Input: part model. Units: mm. Frame: model coordinates. Give positions to 0.01 mm unless a question says otherwise; leave off trailing zeros. Loops run counter-clockwise (first coordinate to the right, second up) from the corner with the lowest first, then second, coordinate; pieces in that order, holes last.
from build123d import *

# Parameters (mm, degrees)
CYLINDER013_R          = 0.565
CYLINDER013_DEPTH      = 5
CYLINDER012_R          = 0.565
CYLINDER012_DEPTH      = 5
CYLINDER008_R          = 0.565
CYLINDER008_DEPTH      = 5
CYLINDER003_R          = 0.565
CYLINDER003_DEPTH      = 5
BOX018_W               = 0.4
BOX018_H               = 1
BOX018_DEPTH           = 1
BOX018_PLACEMENT_ANGLE = 90
BOX001_W               = 0.4
BOX001_H               = 1
BOX001_DEPTH           = 1
BOX001_PLACEMENT_ANGLE = 90
BOX014_W               = 0.4
BOX014_H               = 1
BOX014_DEPTH           = 1
BOX014_PLACEMENT_ANGLE = 90
BOX015_W               = 0.4
BOX015_H               = 1
BOX015_DEPTH           = 1
BOX015_PLACEMENT_ANGLE = 90
BOX017_W               = 0.4
BOX017_H               = 1
BOX017_DEPTH           = 1
BOX016_W               = 0.4
BOX016_H               = 1
BOX016_DEPTH           = 1
BOX013_W               = 0.4
BOX013_H               = 1
BOX013_DEPTH           = 1
BOX_W                  = 0.4
BOX_H                  = 1
BOX_DEPTH              = 1
BOX012_W               = 11
BOX012_H               = 11
BOX012_DEPTH           = 0.3
CHAMFER002_SIZE        = 0.5
CUT010_PLACEMENT_ANGLE = 90


with BuildPart() as cilindro009:
    # Cylinder013 → Cylinder013 (new body)
    with BuildSketch(Plane(origin=(4.2, -4.2, 0), x_dir=(1, 0, 0), z_dir=(0, 0, 1))):
        Circle(CYLINDER013_R)
    extrude(amount=CYLINDER013_DEPTH)


with BuildPart() as cilindro008:
    # Cylinder012 → Cylinder012 (new body)
    with BuildSketch(Plane(origin=(-4.2, -4.2, 0), x_dir=(1, 0, 0), z_dir=(0, 0, 1))):
        Circle(CYLINDER012_R)
    extrude(amount=CYLINDER012_DEPTH)


with BuildPart() as cilindro006:
    # Cylinder008 → Cylinder008 (new body)
    with BuildSketch(Plane(origin=(4.2, 4.2, 0), x_dir=(1, 0, 0), z_dir=(0, 0, 1))):
        Circle(CYLINDER008_R)
    extrude(amount=CYLINDER008_DEPTH)


with BuildPart() as cilindro007:
    # Cylinder003 → Cylinder003 (new body)
    with BuildSketch(Plane(origin=(-4.2, 4.2, 0), x_dir=(1, 0, 0), z_dir=(0, 0, 1))):
        Circle(CYLINDER003_R)
    extrude(amount=CYLINDER003_DEPTH)


with BuildPart() as obj1:
    # Box018 → Box018 (new body)
    with BuildSketch(Plane.XY):
        with Locations((0.2, 0.5)):
            Rectangle(BOX018_W, BOX018_H)
    extrude(amount=BOX018_DEPTH)


with BuildPart() as obj1_1:
    # Box018 placement: moved
    add(obj1.part.moved(Location((6.3, -3, 3))).rotate(Axis((6.3, -3, 3), (0, 0, 1)), BOX018_PLACEMENT_ANGLE))


with BuildPart() as obj2:
    # Box001 → Box001 (new body)
    with BuildSketch(Plane.XY):
        with Locations((0.2, 0.5)):
            Rectangle(BOX001_W, BOX001_H)
    extrude(amount=BOX001_DEPTH)


with BuildPart() as obj2_1:
    # Box001 placement: moved
    add(obj2.part.moved(Location((6.3, 2.5, 3))).rotate(Axis((6.3, 2.5, 3), (0, 0, 1)), BOX001_PLACEMENT_ANGLE))


with BuildPart() as obj3:
    # Box014 → Box014 (new body)
    with BuildSketch(Plane.XY):
        with Locations((0.2, 0.5)):
            Rectangle(BOX014_W, BOX014_H)
    extrude(amount=BOX014_DEPTH)


with BuildPart() as obj3_1:
    # Box014 placement: moved
    add(obj3.part.moved(Location((-5.3, -3, 3))).rotate(Axis((-5.3, -3, 3), (0, 0, 1)), BOX014_PLACEMENT_ANGLE))


with BuildPart() as obj4:
    # Box015 → Box015 (new body)
    with BuildSketch(Plane.XY):
        with Locations((0.2, 0.5)):
            Rectangle(BOX015_W, BOX015_H)
    extrude(amount=BOX015_DEPTH)


with BuildPart() as obj4_1:
    # Box015 placement: moved
    add(obj4.part.moved(Location((-5.3, 2.5, 3))).rotate(Axis((-5.3, 2.5, 3), (0, 0, 1)), BOX015_PLACEMENT_ANGLE))


with BuildPart() as obj5:
    # Box017 → Box017 (new body)
    with BuildSketch(Plane(origin=(3, -6.2, 3), x_dir=(1, 0, 0), z_dir=(0, 0, 1))):
        with Locations((0.2, 0.5)):
            Rectangle(BOX017_W, BOX017_H)
    extrude(amount=BOX017_DEPTH)


with BuildPart() as obj6:
    # Box016 → Box016 (new body)
    with BuildSketch(Plane(origin=(-3, -6.2, 3), x_dir=(1, 0, 0), z_dir=(0, 0, 1))):
        with Locations((0.2, 0.5)):
            Rectangle(BOX016_W, BOX016_H)
    extrude(amount=BOX016_DEPTH)


with BuildPart() as obj7:
    # Box013 → Box013 (new body)
    with BuildSketch(Plane(origin=(3, 5.2, 3), x_dir=(1, 0, 0), z_dir=(0, 0, 1))):
        with Locations((0.2, 0.5)):
            Rectangle(BOX013_W, BOX013_H)
    extrude(amount=BOX013_DEPTH)


with BuildPart() as obj8:
    # Box → Box (new body)
    with BuildSketch(Plane(origin=(-3, 5.2, 3), x_dir=(1, 0, 0), z_dir=(0, 0, 1))):
        with Locations((0.2, 0.5)):
            Rectangle(BOX_W, BOX_H)
    extrude(amount=BOX_DEPTH)


with BuildPart() as obj9:
    # Box012 → Box012 (new body)
    with BuildSketch(Plane(origin=(-5.5, -5.5, 3.6), x_dir=(1, 0, 0), z_dir=(0, 0, 1))):
        with Locations((5.5, 5.5)):
            Rectangle(BOX012_W, BOX012_H)
    extrude(amount=BOX012_DEPTH)

    # Chamfer002
    chamfer002_edges = [obj9.edges().sort_by_distance(p)[0] for p in [
        (-5.5, -5.5, 3.75),
        (-5.5, 5.5, 3.75),
        (5.5, -5.5, 3.75),
        (5.5, 5.5, 3.75),
    ]]
    chamfer(chamfer002_edges, length=CHAMFER002_SIZE)


with BuildPart() as obj9_1:
    # Chamfer002 placement: moved
    add(obj9.part.moved(Location((0, 0, -0.4))))

    # Cut021: cut obj8
    add(obj8.part, mode=Mode.SUBTRACT)

    # Cut022: cut obj7
    add(obj7.part, mode=Mode.SUBTRACT)

    # Cut029: cut obj6
    add(obj6.part, mode=Mode.SUBTRACT)

    # Cut006: cut obj5
    add(obj5.part, mode=Mode.SUBTRACT)

    # Cut005: cut obj4
    add(obj4_1.part, mode=Mode.SUBTRACT)

    # Cut023: cut obj3
    add(obj3_1.part, mode=Mode.SUBTRACT)

    # Cut009: cut obj2
    add(obj2_1.part, mode=Mode.SUBTRACT)

    # Cut003: cut obj1
    add(obj1_1.part, mode=Mode.SUBTRACT)

    # Cut028: cut Cilindro007
    add(cilindro007.part, mode=Mode.SUBTRACT)

    # Cut027: cut Cilindro006
    add(cilindro006.part, mode=Mode.SUBTRACT)

    # Cut004: cut Cilindro008
    add(cilindro008.part, mode=Mode.SUBTRACT)

    # Cut010: cut Cilindro009
    add(cilindro009.part, mode=Mode.SUBTRACT)


with BuildPart() as obj9_2:
    # Cut010 placement: moved
    add(obj9_1.part.moved(Location((0, 1.7, 1.6))).rotate(Axis((0, 1.7, 1.6), (0, 0, 1)), CUT010_PLACEMENT_ANGLE))


solid = obj9_2.part
(1) Pin query (flat end, axial travel): pin 1 Ø1.5 at (x, y) = (-4.2, -2.5) entering from -Z. Return the tip coordinate at first contact, or that it passes through.
Values follow:
pin 1: stops at z = 4.8
(2) Ray query, probe 1 along X at (y, z) = (-2.5, 5) (3 decimals); probe 2 along Y at (x, z) = (4.25, 4.9); probe 3 along Y at (x, z) = (5.25, 4.85). Return the intervals inside material, ascending.
Values follow:
probe 1: x = -5.5 to -4.765, -3.635 to 3.635, 4.765 to 5.5
probe 2: y = -3.8 to -3.06, -1.94 to 5.34, 6.46 to 7.2
probe 3: y = -3.55 to -1.3, -0.9 to 4.7, 5.1 to 6.95
(3) Cut plane A-A (y = 5.9). Return the cut outline in (x, z) (3 decimals), and give its area (3 significant figures).
Values follow:
outline: (-5.5, 4.8) - (-4.765, 4.8) - (-4.765, 5.1) - (-5.5, 5.1) - close; (-3.635, 4.8) - (3.635, 4.8) - (3.635, 5.1) - (-3.635, 5.1) - close; (4.765, 4.8) - (5.5, 4.8) - (5.5, 5.1) - (4.765, 5.1) - close
area: 2.62 mm2
(4) Cut plane C-C (z = 4.95). Count the separate pieces of the cut face and the enclosed holes in it, and give its area (3 significant figures).
Values follow:
separate pieces: 1
enclosed holes: 4
area: 116 mm2
(5) Cut plane B-B (x = 4.2). Return the cut outline in (y, z) (3 decimals), and give its area (3 significant figures).
Values follow:
outline: (-3.8, 4.8) - (-3.065, 4.8) - (-3.065, 5.1) - (-3.8, 5.1) - close; (-1.935, 4.8) - (5.335, 4.8) - (5.335, 5.1) - (-1.935, 5.1) - close; (6.465, 4.8) - (7.2, 4.8) - (7.2, 5.1) - (6.465, 5.1) - close
area: 2.62 mm2
(6) Mould query, pull axis Y, two halves, no side actions, for faces 1 (the cylindrical face through (4.54, 5.45, 4.95)), 2 (the flat face through (0, 2, 5.1)), 3 (the cylindrical face through (-3.86, 5.45, 4.95)). Classes: +Y half, -Y half, draft (parallel to the pull), parting line (faces both ways), or undercut.
Values follow:
face 1: undercut
face 2: draft
face 3: undercut
